Check sheet for the modelled part. Datum: model origin and axes. Units: mm. A direction names the side the tool comes from. Give positions to 0.01 mm unless a question says otherwise; leave off trailing zeros. Loops run counter-clockwise (first coordinate to the right, second up) from the corner with the lowest first, then second, coordinate; pieces in that order, holes last. Notation, with made-up numbers: (-0.5, 59.25) - (55.5, 59.25) arc R25 cw to (55.5, 87.25) - close; hole circle Ø7 at (14, 31). An arc over 180 degrees is marked (long way). Use one line per item in the form item = value.
from build123d import *

# Parameters (mm, degrees)
F0_R      = 15.875
F1_DEPTH  = 5.334
F2_R      = 12.7
F3_DEPTH  = 4.445
F4_R      = 15.875
F5_DEPTH  = 8.255
F6_R      = 12.7
F7_DEPTH  = 4.445
F8_R      = 15.875
F9_DEPTH  = 6.35
F10_R     = 12.7
F11_DEPTH = 48.26


with BuildPart() as f1:
    # F0 (on Front) → F1 (new body)
    with BuildSketch(Plane.XZ):
        Circle(F0_R)
    extrude(amount=F1_DEPTH)

    # F2 (on face) → F3 (join)
    with BuildSketch(Plane.XZ.offset(5.334)):
        Circle(F2_R)
    extrude(amount=F3_DEPTH)

    # F4 (on face) → F5 (join)
    with BuildSketch(Plane.XZ.offset(9.779)):
        Circle(F4_R)
    extrude(amount=F5_DEPTH)

    # F6 (on face) → F7 (join)
    with BuildSketch(Plane.XZ.offset(18.034)):
        Circle(F6_R)
    extrude(amount=F7_DEPTH)

    # F8 (on face) → F9 (join)
    with BuildSketch(Plane.XZ.offset(22.479)):
        Circle(F8_R)
    extrude(amount=F9_DEPTH)

    # F10 (on face) → F11 (join)
    with BuildSketch(Plane.XZ.offset(28.829)):
        Circle(F10_R)
    extrude(amount=F11_DEPTH)


solid = f1.part
Item 1: Gauge pin test, flat ends, axial feed: P1, Ø12, axis at x = -2.5, y = -64, coming from the -Z side; P2, Ø1, axis at x = 4.5, y = -11.5, coming from the +Z side; P3, Ø16, axis at x = 4.5, z = 6, coming from the +Y side; P4, Ø3, axis at y = -57, z = -8.5, coming from the +X side. Record the tip position at first contact, or that the pin passes through.
Answer block:
P1 = -12.7
P2 = 15.36
P3 = 0
P4 = 10.6
Item 2: Section check C-C on y = -49.5. Record the boundary of the cut face in (x, z), then the cut area to 3 significant figures.
Answer block:
outline = circle Ø25.4 at (0, 0)
area = 507 mm2
Item 3: Thickness scan on L1, parallel to Y at x = 11, z = 7; L2, parallel to Z at x = -8.5, y = -63.5; L3, parallel to Z at x = 9.5, y = -9.5. Record the ranges inside material, lowest first.
Answer block:
L1 = -28.83 to -22.48, -18.03 to -9.78, -5.33 to 0
L2 = -9.44 to 9.44
L3 = -8.43 to 8.43
Item 4: Section check B-B on z = 7.5. Record the boundary of the cut face in (x, y), then the cut area to 3 significant figures.
Answer block:
outline = (-13.99, -28.83) - (-10.25, -28.83) - (-10.25, -77.09) - (10.25, -77.09) - (10.25, -28.83) - (13.99, -28.83) - (13.99, -22.48) - (10.25, -22.48) - (10.25, -18.03) - (13.99, -18.03) - (13.99, -9.78) - (10.25, -9.78) - (10.25, -5.33) - (13.99, -5.33) - (13.99, 0) - (-13.99, 0) - (-13.99, -5.33) - (-10.25, -5.33) - (-10.25, -9.78) - (-13.99, -9.78) - (-13.99, -18.03) - (-10.25, -18.03) - (-10.25, -22.48) - (-13.99, -22.48) - close
area = 1,730 mm2
Item 5: Mould release check, pull along Y, two halves, no side actions. Record for faces 1 (the face through (-2.75, -52.62, -12.4)), 2 (the face through (-2.75, -7.53, -12.4)), 3 (the face through (0, 0, 0)), 4 (the face through (-7, -28.829, 11)): released by +Y, released by -Y, zero draft, split by the parting line, or undercut.
Answer block:
face_1 = zero draft
face_2 = undercut
face_3 = released by +Y
face_4 = released by -Y
Item 6: Access from +Z, -Z, +X, -X, +Y, -Y to the whole of each face (thin tool, end or side, straight path). Record for faces 5 (the face through (-3.441, -13.849, -15.497)), 6 (the face through (-2.75, -20.23, -12.4)).
Answer block:
face_5 = +Y, -Y
face_6 = none
Item 7: Section check A-A on x = 0. Record the boundary of the cut face in (y, z) (3 decimals), then the cut area to 3 significant figures.
Answer block:
outline = (-77.089, -12.7) - (-28.829, -12.7) - (-28.829, -15.875) - (-22.479, -15.875) - (-22.479, -12.7) - (-18.034, -12.7) - (-18.034, -15.875) - (-9.779, -15.875) - (-9.779, -12.7) - (-5.334, -12.7) - (-5.334, -15.875) - (0, -15.875) - (0, 15.875) - (-5.334, 15.875) - (-5.334, 12.7) - (-9.779, 12.7) - (-9.779, 15.875) - (-18.034, 15.875) - (-18.034, 12.7) - (-22.479, 12.7) - (-22.479, 15.875) - (-28.829, 15.875) - (-28.829, 12.7) - (-77.089, 12.7) - close
area = 2,080 mm2
